Read the model definition and answer for the solid it produces. Units are mm, in the model's axes. A direction names the side the tool comes from. Coordinates: 2 decimals unless noted, no trailing zeros. Write each loop counter-clockwise with the first axis right and the second up, starting at its lowest first coordinate (ties: lowest second). Pieces come first, ordered by that corner, then holes. Notation, with made-up numbers: (85.5, -20) - (100.5, -20) arc R24 cw to (100.5, -3) - close; hole circle Ø3 at (34, -1). An arc over 180 degrees is marked (long way). Return JSON: item names as keys, results as strings.
```python
from build123d import *

# Parameters (mm, degrees)
CUT_EXTRUDE1_DEPTH = 4


with BuildPart() as part:
    # Sketch1 → Revolve1 (revolve)
    with BuildSketch(Plane.XY):
        Polygon((0, 0), (14, 0), (14, 4), (13.5, 4.5), (10, 4.5), (10, 2.5), (5, 2.5), (5, 2), (0.5, 2), (0, 1.5), align=None)
    revolve(axis=Axis((0, 0, 0), (1, 0, 0)))

    # Sketch2 → Cut-Extrude1 (cut)
    with BuildSketch(Plane(origin=(14, 0, 0), x_dir=(0, 0, -1), z_dir=(1, 0, 0))):
        Polygon((1.443375673, 0), (0.721687836, 1.25), (-0.721687836, 1.25), (-1.443375673, 0), (-0.721687836, -1.25), (0.721687836, -1.25), align=None)
    extrude(amount=-CUT_EXTRUDE1_DEPTH, mode=Mode.SUBTRACT)


solid = part.part
```
(1) A cutting plane is placed at C-C (x = 5.25). Determine the outline of the cut face in (y, z).
Answer:
{"outline": "circle Ø5 at (0, 0)"}
(2) Straight lines are drawn through the part: line 1 (X direction, y = -1.5, z = -1.5); line 2 (X direction, y = 1, z = 3.5); line 3 (Y direction, x = 13.25, z = 1.25). For each, find the intervals that lie inside material, in ascending order. Write a range as from..to.
Answer:
{"line 1": "5..14", "line 2": "10..14", "line 3": "-4.32..-0.33, 0.33..4.32"}
(3) Flat-ended cylindrical pins translate along their axes: P1, Ø0.8, axis at y = 0.5, z = -0.5, coming from the +X side; P2, Ø1.5, axis at y = -3.5, z = 1, coming from the -X side; P3, Ø1.5, axis at x = 12, y = 2, coming from the +Z side. Find the tip coordinate at first contact, or state that the pin passes through.
Answer:
{"P1": "x = 10", "P2": "x = 10", "P3": "z = 4.32"}
(4) Determine the mould class of faces 1 (the face through (5, -1, 2)), 2 (the face through (12.028, 0.616, -1.088)), 3 (the face through (12.03, 0.63, 1.08)), 4 (the face through (7.46, -0.54, -2.44)) for opening direction Y: +Y half, -Y half, draft (parallel to the pull), parting line (faces both ways), or undercut.
Answer:
{"face 1": "draft", "face 2": "undercut", "face 3": "undercut", "face 4": "parting line"}
(5) A cutting plane is placed at B-B (x = 12). Determine the outline of the cut face in (y, z), and give its area (3 significant figures).
Answer:
{"outline": "circle Ø9 at (0, 0); hole (-1.25, -0.72) - (0, -1.44) - (1.25, -0.72) - (1.25, 0.72) - (0, 1.44) - (-1.25, 0.72) - close", "area": "58.2 mm²"}
(6) A cutting plane is placed at A-A (z = 0). Determine the outline of the cut face in (x, y), and give its area (3 significant figures).
Answer:
{"outline": "(0, -1.5) - (0.5, -2) - (5, -2) - (5, -2.5) - (10, -2.5) - (10, -4.5) - (13.5, -4.5) - (14, -4) - (14, -1.25) - (10, -1.25) - (10, 1.25) - (14, 1.25) - (14, 4) - (13.5, 4.5) - (10, 4.5) - (10, 2.5) - (5, 2.5) - (5, 2) - (0.5, 2) - (0, 1.5) - close", "area": "70.5 mm²"}
(7) Which of the six approach directions +Z, -Z, +X, -X, +Y, -Y give full straight-line access (tool end or side, diameter ignored) to faces 5 (the face through (12, -1.25, 0)), 6 (the face through (14, -2, 0)), 7 (the face through (10, 2, -2))?
Answer:
{"face 5": "+X", "face 6": "+Z, -Z, +X, +Y, -Y", "face 7": "-X"}
